from build123d import *

# Parameters (mm, degrees)
SKETCH1_R           = 70
BOSS_EXTRUDE1_DEPTH = 7
SKETCH3_R           = 1
CUT_EXTRUDE1_DEPTH  = 12
CIRPATTERN1_COUNT   = 4
BOSS_EXTRUDE2_DEPTH = 12
SKETCH5_R           = 1.375
CUT_EXTRUDE2_DEPTH  = 12
SKETCH6_R           = 1.375
CUT_EXTRUDE3_DEPTH  = 12
CUT_EXTRUDE4_DEPTH  = 12


with BuildPart() as part:
    # Sketch1 → Boss-Extrude1 (new body)
    with BuildSketch(Plane.XY):
        Circle(SKETCH1_R)
    extrude(amount=BOSS_EXTRUDE1_DEPTH)

    # Sketch3 → Cut-Extrude1 (cut)
    with BuildSketch(Plane(origin=(0, 70, 0), x_dir=(1, 0, 0), z_dir=(0, 1, 0))):
        with Locations(Location((0, -3.5, 0), (0, 0, 270))):
            Circle(SKETCH3_R)
    cut_extrude1 = extrude(amount=-CUT_EXTRUDE1_DEPTH, mode=Mode.SUBTRACT)

    # CirPattern1: Cut-Extrude1 ×4 about axis
    cirpattern1_axis = Axis((0, 0, 0), (0, 0, 1))
    for i in range(1, CIRPATTERN1_COUNT):
        add(cut_extrude1.rotate(cirpattern1_axis, i * 360 / CIRPATTERN1_COUNT), mode=Mode.SUBTRACT)

    # Sketch4 → Boss-Extrude2 (add)
    with BuildSketch(Plane(origin=(0, 0, 0), x_dir=(-1, 0, 0), z_dir=(0, 0, -1))):
        Polygon((31.875552268, 8.541028488), (48.296291314, 12.940952255), (45.708100863, 22.600210518), (40.878471732, 21.306115293), (42.690205048, 14.544634508), (31.099095132, 11.438805967), align=None)
        Polygon((56.785555994, -18.741414847), (51.955926862, -20.035510073), (50.144193547, -13.274029289), (38.553083631, -16.37985783), (37.776626496, -13.482080351), (54.197365543, -9.082156584), align=None)
    boss_extrude2 = extrude(amount=BOSS_EXTRUDE2_DEPTH)

    # Mirror1: Boss-Extrude2 across plane
    add(boss_extrude2.mirror(Plane(origin=(0, 0, 0), x_dir=(0, 0, 1), z_dir=(1, 0, 0))))

    # Sketch5 → Cut-Extrude2 (cut)
    with BuildSketch(Plane(origin=(-48.296291314, 12.940952255, 0), x_dir=(0, 0, 1), z_dir=(-0.9659258262890689, 0.2588190451025187, 0))):
        with Locations(Location((-6.2, -25.4, 0), (0, 0, 270))):
            Circle(SKETCH5_R)
    cut_extrude2 = extrude(amount=-CUT_EXTRUDE2_DEPTH, mode=Mode.SUBTRACT)

    # Sketch6 → Cut-Extrude3 (cut)
    with BuildSketch(Plane(origin=(-48.296291314, 12.940952255, 0), x_dir=(0, 0, 1), z_dir=(-0.9659258262890691, 0.2588190451025179, 0))):
        with Locations(Location((-6.2, 2.6, 0), (0, 0, 270))):
            Circle(SKETCH6_R)
    cut_extrude3 = extrude(amount=-CUT_EXTRUDE3_DEPTH, mode=Mode.SUBTRACT)

    # Mirror2: Cut-Extrude2, Cut-Extrude3 across plane
    add(cut_extrude2.mirror(Plane(origin=(0, 0, 0), x_dir=(0, 0, 1), z_dir=(1, 0, 0))), mode=Mode.SUBTRACT)
    add(cut_extrude3.mirror(Plane(origin=(0, 0, 0), x_dir=(0, 0, 1), z_dir=(1, 0, 0))), mode=Mode.SUBTRACT)

    # Sketch7 → Cut-Extrude4 (cut)
    with BuildSketch(Plane(origin=(0, 0, 0), x_dir=(-1, 0, 0), z_dir=(0, 0, -1))):
        with BuildLine():
            ThreePointArc((-57.113972469, -40.472140403), (-41.814961007, -44.896509701), (-36.315733397, -59.842856782))
            ThreePointArc((-36.315733397, -59.842856782), (-47.708318434, -51.224177419), (-57.113972469, -40.472140403))
        make_face()
    extrude(amount=-CUT_EXTRUDE4_DEPTH, mode=Mode.SUBTRACT)


solid = part.part
For this review, take the finished solid that the model builds, in its own axes (mm). A direction names the side the tool comes from. Give positions to 0.01 mm unless a question says otherwise; leave off trailing zeros. Order: outer loops, then holes, each group sorted by start corner. A loop starts at its lowest first (then second) coordinate and runs counter-clockwise, first axis right, second up. Notation, with made-up numbers: M 68,57.25 L 78,57.25 A10 ccw 78,72.25 Z; hole C -20.75,79 d6. An arc over 180 degrees is marked long. Answer in a Markdown table with one row per item. Add a question column.
(1) Wall thickness on probe 1 along Z at (x, y) = (0, 66); probe 2 along Z at (x, y) = (-49.5, 0); probe 3 along X at (y, z) = (-64, 4): over which ranges is each line inside the solid? List them lowest first. Write a range as [from, to].
(2) Consider section B-B on y = -3. State the section outline as (x, z) points, and give its area (3 significant figures).
(3) For pin 1 (5 mm diameter, centred on y = -45, z = -0.5, fed in from +X); pin 2 (1.2 mm diameter, centred on y = 0, z = 3.5, fed in from -X); pin 3 (1 mm diameter, centred on y = 43.5, z = 3, fed in from -X); pin 4 (1 mm diameter, centred on y = -7.5, z = -9.5, fed in from -X), all flat-tipped, find the tip position at first contact; note any pin that passes through.
(4) Consider section C-C on x = 12. State the section outline as (y, z) points, and give its area (3 significant figures).
(5) For faces 4 (the face through (-43.327, 21.962, -5.916)), 5 (the face through (-55.473, -13.844, -5.916)), 6 (the face through (45.872, -11.313, -5.916)), 7 (the face through (-43.14, -15.15, -5.92)), list the 3-axis set-ups (+Z, -Z, +X, -X, +Y, -Y) from which the entire face can be reached by the end or side of a thin tool; tool diameter is ignored.
(6) Mouldability with a two-part tool opening along Y and no side actions: class faces 1 (the face through (-54.4, -19.38, -5.92)), 2 (the face through (55.473, -13.844, -5.916)), 3 (the face through (41.772, 17.973, -5.916)) as +Y half, -Y half, draft (parallel to the pull), parting line (faces both ways), or undercut.
(7) Consider section A-A on x = -33.5. State the section outline as (y, z) points.
Evaluation:
| question | item | result |
|---|---|---|
| 1 | probe 1 | z = [0, 2.5], [4.5, 7] |
| 1 | probe 2 | z = [0, 7] |
| 1 | probe 3 | x = [-28.35, -0.87], [0.87, 28.35] |
| 2 | outline | M -69.94,0 L 69.94,0 L 69.94,7 L -69.94,7 Z |
| 2 | area | 979 mm^2 |
| 3 | pin 1 | stops at x = 44.98 |
| 3 | pin 2 | stops at x = -58 |
| 3 | pin 3 | stops at x = -55.24 |
| 3 | pin 4 | passes through |
| 4 | outline | M -68.96,0 L 68.96,0 L 68.96,7 L -68.96,7 Z |
| 4 | area | 965 mm^2 |
| 5 | face 4 | -Z, +Y |
| 5 | face 5 | -Z, -X, +Y |
| 5 | face 6 | -Z |
| 5 | face 7 | -Z, -Y |
| 6 | face 1 | -Y half |
| 6 | face 2 | +Y half |
| 6 | face 3 | undercut |
| 7 | outline | M -61.46,0 L 8.98,0 L 8.98,-12 L 12.08,-12 L 12.08,0 L 61.46,0 L 61.46,7 L -61.46,7 Z |
